For this review, take the finished solid that the model builds, in its own axes (mm). A direction names the side the tool comes from. Coordinates: 2 decimals unless noted, no trailing zeros. Write each loop counter-clockwise with the first axis right and the second up, starting at its lowest first coordinate (ties: lowest second). Pieces come first, ordered by that corner, then holes.
```python
from build123d import *

# Parameters (mm, degrees)
PAD_DEPTH       = 26
PAD001_DEPTH    = 26
SKETCH002_W     = 36
SKETCH002_H     = 20
POCKET_DEPTH    = 17.5
PAD002_DEPTH    = 26
SKETCH004_R     = 1.8
POCKET001_DEPTH = 40.061
SKETCH005_R     = 6
POCKET002_DEPTH = 2.501
SKETCH006_W     = 2
SKETCH006_H     = 1.2
PAD003_DEPTH    = 2.5
FILLET_R        = 0.49


with BuildPart() as part:
    # Sketch → Pad (new body)
    with BuildSketch(Plane.XY):
        Polygon((0, 0), (0, 38.5), (-2.5, 38.5), (-2.5, 2.5), (-20, 2.5), (-20, 0), align=None)
    extrude(amount=PAD_DEPTH)

    # Sketch001 (on Face7 of Pad) → Pad001 (join)
    with BuildSketch(Plane(origin=(0, 0, 0), x_dir=(1, 0, 0), z_dir=(0, 0, -1))):
        Polygon((-20, -2.5), (-2.5, -38.5), (-2.5, -2.5), align=None)
    extrude(amount=-PAD001_DEPTH)

    # Sketch002 (on Face6 of Pad001) → Pocket (cut)
    with BuildSketch(Plane(origin=(-20, 0, 0), x_dir=(0, -1, 0), z_dir=(-1, 0, 0))):
        with Locations((-20.5, 13)):
            Rectangle(SKETCH002_W, SKETCH002_H)
    extrude(amount=-POCKET_DEPTH, mode=Mode.SUBTRACT)

    # Sketch003 (on Face4 of Pocket) → Pad002 (join)
    with BuildSketch(Plane(origin=(0, 0, 0), x_dir=(1, 0, 0), z_dir=(0, 0, -1))):
        Polygon((-14.74, 0), (-5.26, 0), (-7.06, 1.56), (-12.94, 1.56), align=None)
    extrude(amount=-PAD002_DEPTH)

    # Sketch004 (on Face16 of Pad002) → Pocket001 (cut, through all)
    with BuildSketch(Plane.XZ.offset(1.56)):
        with Locations((-10, 18.286)):
            Circle(SKETCH004_R)
        with Locations((-10, 7.714)):
            Circle(SKETCH004_R)
    extrude(amount=-POCKET001_DEPTH, mode=Mode.SUBTRACT)

    # Sketch005 (on Face8 of Pocket001) → Pocket002 (cut, through all)
    with BuildSketch(Plane(origin=(-2.5, 0, 0), x_dir=(0, -1, 0), z_dir=(-1, 0, 0))):
        with Locations((-22.5, 13)):
            Circle(SKETCH005_R)
    extrude(amount=-POCKET002_DEPTH, mode=Mode.SUBTRACT)

    # Sketch006 (on Face1 of Pocket002) → Pad003 (join)
    with BuildSketch(Plane.YZ):
        with Locations((28.869925, 13)):
            Rectangle(SKETCH006_W, SKETCH006_H)
    extrude(amount=-PAD003_DEPTH)

    # Fillet
    fillet_edges = [part.edges().sort_by_distance(p)[0] for p in [
        (-1.25, 27.869925, 12.4),
        (-1.25, 27.869925, 13.6),
    ]]
    fillet(fillet_edges, radius=FILLET_R)


solid = part.part
```
Q1. Add section B-B (x = -9.25). State the section outline as (y, z) points.
Ans:
outline: (-1.56, 0) - (24.61, 0) - (24.61, 3) - (2.5, 3) - (2.5, 6.08) - (-1.56, 6.08) - close; (-1.56, 9.35) - (2.5, 9.35) - (2.5, 16.65) - (-1.56, 16.65) - close; (-1.56, 19.92) - (2.5, 19.92) - (2.5, 23) - (24.61, 23) - (24.61, 26) - (-1.56, 26) - close
Q2. Tool access review of faces 1 (the flat face through (-7, 13, 3)), 2 (the flat face through (-8, 14, 26)), 3 (the flat face through (-3, 0, 13)): name each direction out of +Z, -Z, +X, -X, +Y, -Y from which nothing blocks a thin tool from reaching the whole face with its end or side.
Ans:
face 1: -X, +Y
face 2: +Z, +X, -X, +Y, -Y
face 3: +Z, -Z, +X, -Y
Q3. Add section C-C (x = -14.25). State the section outline as (y, z) points, then the cut area to 3 significant figures.
Ans:
outline: (-0.42, 0) - (14.33, 0) - (14.33, 3) - (2.5, 3) - (2.5, 23) - (14.33, 23) - (14.33, 26) - (-0.42, 26) - close
area: 147 mm2
Q4. Clearance check with flat-ended pins moving along their axes: pin 1 Ø3 at (x, z) = (-14, 20) entering from +Y; pin 2 Ø4 at (x, z) = (-16, 9.5) entering from -Y; pin 3 Ø1.6 at (x, z) = (-18, 13) entering from -Y. State where each tip first meets the part, or that it passes through.
Ans:
pin 1: stops at y = 2.5
pin 2: stops at y = -0.64
pin 3: stops at y = 0
Q5. Add section A-A (y = 21). State the section outline as (x, z) points.
Ans:
outline: (-11.01, 0) - (0, 0) - (0, 7.19) - (-2.5, 7.19) - (-2.5, 3) - (-11.01, 3) - close; (-11.01, 23) - (-2.5, 23) - (-2.5, 18.81) - (0, 18.81) - (0, 26) - (-11.01, 26) - close
Q6. Draft analysis for pull direction X (two halves, no side actions). For faces 4 (the cylindrical face through (-11.8, 0.44, 7.79)), 5 (the flat face through (-2.5, 16, 13)), 6 (the flat face through (-17, 0, 13)), state which applies: +X half, -X half, draft (parallel to the pull), parting line (faces both ways), or undercut.
Ans:
face 4: undercut
face 5: -X half
face 6: draft
Q7. For probe 1 along Z at (x, y) = (-10, 0.95); probe 2 along Z at (x, y) = (-6, 22.5); probe 3 along Y at (x, z) = (-7.5, 21.5), list the stretches that pass through material, from the lowest coordinate up.
Ans:
probe 1: z = 0 to 5.91, 9.51 to 16.49, 20.09 to 26
probe 2: z = 0 to 3, 23 to 26
probe 3: y = -1.56 to 2.5
Q8. Add section D-D (y = 31). State the section outline as (x, z) points.
Ans:
outline: (-6.15, 0) - (0, 0) - (0, 26) - (-6.15, 26) - (-6.15, 23) - (-2.5, 23) - (-2.5, 3) - (-6.15, 3) - close
